from build123d import *

# Parameters (mm, degrees)
SKETCH1_W                 = 278
SKETCH1_H                 = 260
BOSS_EXTRUDE1_DEPTH       = 60.5
SKETCH2_R                 = 90.5
CUT_EXTRUDE2_DEPTH        = 42
SKETCH3_R                 = 41.5
CUT_EXTRUDE3_DEPTH        = 386.414387381
SKETCH4_R                 = 99.95
SKETCH4_R_2               = 95.05
CUT_EXTRUDE5_DEPTH        = 2.95
SKETCH6_W                 = 278
SKETCH6_H                 = 260
SKETCH6_W_2               = 250
SKETCH6_H_2               = 232
CUT_EXTRUDE6_DEPTH        = 39
SKETCH7_W                 = 259.8
SKETCH7_H                 = 241.8
SKETCH7_W_2               = 250
SKETCH7_H_2               = 232
CUT_EXTRUDE7_DEPTH        = 41.95
F_8_0MM_DOWEL_HOLE1_D     = 8
F_8_0MM_DOWEL_HOLE1_DEPTH = 15
F_8_0MM_DOWEL_HOLE1_TIP   = 2.403442476
SKETCH10_R                = 3
CUT_EXTRUDE8_DEPTH        = 59


with BuildPart() as part:
    # Sketch1 → Boss-Extrude1 (new body)
    with BuildSketch(Plane.XY):
        with Locations((139, 130)):
            Rectangle(SKETCH1_W, SKETCH1_H)
    extrude(amount=BOSS_EXTRUDE1_DEPTH)

    # Sketch2 → Cut-Extrude2 (cut)
    with BuildSketch(Plane.XY):
        with Locations(Location((127.7, 130, 0), (0, 0, 180))):
            Circle(SKETCH2_R)
    extrude(amount=CUT_EXTRUDE2_DEPTH, mode=Mode.SUBTRACT)

    # Sketch3 → Cut-Extrude3 (cut, through all)
    with BuildSketch(Plane.XY):
        with Locations((127.7, 130)):
            Circle(SKETCH3_R)
    extrude(amount=CUT_EXTRUDE3_DEPTH, mode=Mode.SUBTRACT)

    # Sketch4 → Cut-Extrude5 (cut)
    with BuildSketch(Plane.XY):
        with Locations((127.7, 130)):
            Circle(SKETCH4_R)
        with Locations((127.7, 130)):
            Circle(SKETCH4_R_2, mode=Mode.SUBTRACT)
    extrude(amount=CUT_EXTRUDE5_DEPTH, mode=Mode.SUBTRACT)

    # Sketch6 → Cut-Extrude6 (cut)
    with BuildSketch(Plane.XY.offset(60.5)):
        with Locations((139, 130)):
            Rectangle(SKETCH6_W, SKETCH6_H)
        with Locations((139, 130)):
            Rectangle(SKETCH6_W_2, SKETCH6_H_2, mode=Mode.SUBTRACT)
    extrude(amount=-CUT_EXTRUDE6_DEPTH, mode=Mode.SUBTRACT)

    # Sketch7 → Cut-Extrude7 (cut)
    with BuildSketch(Plane.XY.offset(60.5)):
        with Locations((139, 130)):
            Rectangle(SKETCH7_W, SKETCH7_H)
        with Locations((139, 130)):
            Rectangle(SKETCH7_W_2, SKETCH7_H_2, mode=Mode.SUBTRACT)
    extrude(amount=-CUT_EXTRUDE7_DEPTH, mode=Mode.SUBTRACT)

    # Ø8.0mm Dowel Hole1
    with Locations(Plane(origin=(0, 0, 0), x_dir=(-1, 0, 0), z_dir=(0, 0, -1))):
        with Locations((-181.45, 223.097730907), (-77.93104653, 225.285367557), (-20.2, 130), (-73.95, 36.902269093), (-181.45, 36.902269093), (-235.2, 130)):
            Hole(F_8_0MM_DOWEL_HOLE1_D / 2, depth=F_8_0MM_DOWEL_HOLE1_DEPTH)
            with Locations((0, 0, -(F_8_0MM_DOWEL_HOLE1_DEPTH + F_8_0MM_DOWEL_HOLE1_TIP / 2))):  # 118° drill point
                Cone(0, F_8_0MM_DOWEL_HOLE1_D / 2, F_8_0MM_DOWEL_HOLE1_TIP, mode=Mode.SUBTRACT)

    # Sketch10 → Cut-Extrude8 (cut)
    with BuildSketch(Plane(origin=(0, 0, 0), x_dir=(1, 0, 0), z_dir=(0, 1, 0))):
        with Locations(Location((127.7, -9, 0), (0, 0, 90))):
            Circle(SKETCH10_R)
    extrude(amount=CUT_EXTRUDE8_DEPTH, mode=Mode.SUBTRACT)


solid = part.part
Source: CAD feature listing. Evaluate the final solid. Frame: model axes, mm. A direction names the side the tool comes from. Round coordinates to 2 decimals unless told otherwise and drop trailing zeros. Loops run counter-clockwise (first coordinate to the right, second up) from the corner with the lowest first, then second, coordinate; pieces in that order, holes last. Notation, with made-up numbers: (-1.5, 15) - (30.5, 15) arc R25 ccw to (30.5, 52) - close; hole circle Ø9 at (-38.5, 48). An arc over 180 degrees is marked (long way). Write item = value, one per line. Start each with the question number.
(1) Section query D-D, the plane y = 78. Output: boundary loops of the cut face in (x, z).
(2) Section query B-B, the plane z = 51. Output: boundary loops of the cut face in (x, y).
(3) Ray query, line 1 along X through (y, z) = (223, 21); line 2 along Y through (x, z) = (127, 19); line 3 along Y through (x, z) = (20.2, 7.5). Return the intervals inside material, ascending. Write a range as from..to.
(4) Section query C-C, the plane x = 100. Output: boundary loops of the cut face in (y, z), plus the area to 3 significant figures.
(5) Pull-direction query (Y, two-part tool) for faces 1 (the face through (165, 157, 60.5)), 2 (the face through (137, 0, 11)), 3 (the face through (114.7, 229.1, 1.5)); classes: +Y half, -Y half, draft (parallel to the pull), parting line (faces both ways), or undercut.
(6) Set-up query: faces 4 (the face through (216, 93, 2.95)), 5 (the face through (124.726, 19.499, 9.391)), 6 (the face through (0, 128, 11)), 7 (the face through (128, 5, 21.5)). Return all of +Z, -Z, +X, -X, +Y, -Y with unobstructed straight access to the full face (end or side cutting, diameter ignored); none if empty.
(7) Section query A-A, the plane y = 109.5. Output: boundary loops of the cut face in (x, z), plus the area to 3 significant figures.
(8) Pin query (flat end, axial travel): pin 1 (5.5 mm diameter, centred on x = 127.7, z = 9, fed in from -Y); pin 2 (7 mm diameter, centred on x = 235.2, y = 130, fed in from -Z); pin 3 (12.5 mm diameter, centred on y = 136.5, z = 43, fed in from +X). Return the tip coordinate at first contact, or that it passes through.
Conclusion:
q1.outline = (0, 0) - (42.34, 0) - (42.34, 2.95) - (48.14, 2.95) - (48.14, 0) - (53.63, 0) - (53.63, 42) - (201.77, 42) - (201.77, 0) - (207.26, 0) - (207.26, 2.95) - (213.06, 2.95) - (213.06, 0) - (278, 0) - (278, 21.5) - (268.9, 21.5) - (268.9, 18.55) - (264, 18.55) - (264, 60.5) - (14, 60.5) - (14, 18.55) - (9.1, 18.55) - (9.1, 21.5) - (0, 21.5) - close
q2.outline = (14, 14) - (264, 14) - (264, 246) - (14, 246) - close; hole circle Ø83 at (127.7, 130)
q3.line_1 = 0..9.1, 14..264, 268.9..278
q3.line_2 = 0..9.1, 14..39.5, 220.5..246, 250.9..260
q3.line_3 = 0..126, 134..260
q4.outline = (0, 0) - (33.97, 0) - (33.97, 2.95) - (39.08, 2.95) - (39.08, 0) - (43.84, 0) - (43.84, 42) - (99.1, 42) - (99.1, 60.5) - (14, 60.5) - (14, 18.55) - (9.1, 18.55) - (9.1, 21.5) - (0, 21.5) - close; (160.9, 42) - (216.16, 42) - (216.16, 0) - (220.92, 0) - (220.92, 2.95) - (226.03, 2.95) - (226.03, 0) - (260, 0) - (260, 21.5) - (250.9, 21.5) - (250.9, 18.55) - (246, 18.55) - (246, 60.5) - (160.9, 60.5) - close
q4.area = 6,200 mm2
q5.face_1 = draft
q5.face_2 = -Y half
q5.face_3 = undercut
q6.face_4 = -Z
q6.face_5 = -Y
q6.face_6 = +Z, -Z, -X, +Y, -Y
q6.face_7 = +Z
q7.outline = (0, 0) - (29.87, 0) - (29.87, 2.95) - (34.89, 2.95) - (34.89, 0) - (39.55, 0) - (39.55, 42) - (91.62, 42) - (91.62, 60.5) - (14, 60.5) - (14, 18.55) - (9.1, 18.55) - (9.1, 21.5) - (0, 21.5) - close; (163.78, 42) - (215.85, 42) - (215.85, 0) - (220.51, 0) - (220.51, 2.95) - (225.53, 2.95) - (225.53, 0) - (278, 0) - (278, 21.5) - (268.9, 21.5) - (268.9, 18.55) - (264, 18.55) - (264, 60.5) - (163.78, 60.5) - close
q7.area = 6,930 mm2
q8.pin_1 = 220.46
q8.pin_2 = 15.3
q8.pin_3 = 264
